```python
from build123d import *

# Parameters (mm, degrees)
SKETCH_1_R                  = 15
EXTRUDE_1_DEPTH             = 6.1
SKETCH_1_3_R                = 12.5
EXTRUDE_2_DEPTH             = 10
SKETCH_1_4_R                = 21
EXTRUDE_3_DEPTH             = 4
EXTRUDE_START               = 4
SKETCH_1_6_R                = 16.2
EXTRUDE_4_DEPTH             = 0.5
HOLE_WIZARD_M3_1_AT_2_COUNT = 2
HOLE_WIZARD_M3_1_AT_2_PITCH = 25.455844123
HOLE_WIZARD_M3_1_AT_3_COUNT = 2
HOLE_WIZARD_M3_1_AT_3_PITCH = 36
HOLE_WIZARD_M3_1_AT_4_COUNT = 2
HOLE_WIZARD_M3_1_AT_4_PITCH = 25.455844123
HOLE_WIZARD_M3_2_AT_2_COUNT = 2
HOLE_WIZARD_M3_2_AT_2_PITCH = 24
HOLE_WIZARD_M3_2_AT_3_COUNT = 2
HOLE_WIZARD_M3_2_AT_3_PITCH = 24
HOLE_WIZARD_M3_2_AT_4_COUNT = 2
HOLE_WIZARD_M3_2_AT_4_PITCH = 33.941125497
M5X0_8_1_D                  = 5
PATTERN_CIRCULAR_1_COUNT    = 6
CUT_EXTRUDE_START           = 4
SKETCH_5_R                  = 3.15
CUT_EXTRUDE_3_DEPTH         = 2.1


with BuildPart() as part:
    # ｽｹｯﾁ1 → ﾎﾞｽ - 押し出し1 (new body)
    with BuildSketch(Plane.XY):
        Circle(SKETCH_1_R)
    extrude(amount=EXTRUDE_1_DEPTH)

    # ｽｹｯﾁ1<3> → ﾎﾞｽ - 押し出し2 (add)
    with BuildSketch(Plane.XY):
        Circle(SKETCH_1_3_R)
    extrude(amount=EXTRUDE_2_DEPTH)

    # ｽｹｯﾁ1<4> → ﾎﾞｽ - 押し出し3 (add)
    with BuildSketch(Plane.XY):
        Circle(SKETCH_1_4_R)
    extrude(amount=EXTRUDE_3_DEPTH)

    # ｽｹｯﾁ1<6> → ﾎﾞｽ - 押し出し4 (add)
    with BuildSketch(Plane.XY.offset(EXTRUDE_START)):
        Circle(SKETCH_1_6_R)
    extrude(amount=EXTRUDE_4_DEPTH)

    # ｽｹｯﾁ2 → M3 丸皿ねじ用皿穴1 (revolve, cut)
    with BuildSketch(Plane(origin=(0, 18, 4), x_dir=(0, -1, 0), z_dir=(1, 0, 0))):
        Polygon((0, 0), (0, 4), (1.6, 4), (1.6, 1.55), (3.15, 0), align=None)
    hole_wizard_m3_1 = revolve(axis=Axis((0, 18, 10.35), (0, 0, -1)), mode=Mode.SUBTRACT)

    # M3 丸皿ねじ用皿穴1 at 2: M3 丸皿ねじ用皿穴1 ×2
    with Locations(*[Vector(-0.7071067811865476, -0.7071067811865476, 0) * (i * HOLE_WIZARD_M3_1_AT_2_PITCH) for i in range(1, HOLE_WIZARD_M3_1_AT_2_COUNT)]):
        add(hole_wizard_m3_1, mode=Mode.SUBTRACT)

    # M3 丸皿ねじ用皿穴1 at 3: M3 丸皿ねじ用皿穴1 ×2
    with Locations(*[(0, -i * HOLE_WIZARD_M3_1_AT_3_PITCH, 0) for i in range(1, HOLE_WIZARD_M3_1_AT_3_COUNT)]):
        add(hole_wizard_m3_1, mode=Mode.SUBTRACT)

    # M3 丸皿ねじ用皿穴1 at 4: M3 丸皿ねじ用皿穴1 ×2
    with Locations(*[Vector(0.7071067811865415, -0.7071067811865536, 0) * (i * HOLE_WIZARD_M3_1_AT_4_PITCH) for i in range(1, HOLE_WIZARD_M3_1_AT_4_COUNT)]):
        add(hole_wizard_m3_1, mode=Mode.SUBTRACT)

    # ｽｹｯﾁ8 → M3 丸皿ねじ用皿穴2 (revolve, cut)
    with BuildSketch(Plane(origin=(-12, 12, 4), x_dir=(0, -1, 0), z_dir=(1, 0, 0))):
        Polygon((0, 0), (0, 4), (1.6, 4), (1.6, 1.55), (3.15, 0), align=None)
    hole_wizard_m3_2 = revolve(axis=Axis((-12, 12, 10.35), (0, 0, -1)), mode=Mode.SUBTRACT)

    # M3 丸皿ねじ用皿穴2 at 2: M3 丸皿ねじ用皿穴2 ×2
    with Locations(*[(i * HOLE_WIZARD_M3_2_AT_2_PITCH, 0, 0) for i in range(1, HOLE_WIZARD_M3_2_AT_2_COUNT)]):
        add(hole_wizard_m3_2, mode=Mode.SUBTRACT)

    # M3 丸皿ねじ用皿穴2 at 3: M3 丸皿ねじ用皿穴2 ×2
    with Locations(*[(0, -i * HOLE_WIZARD_M3_2_AT_3_PITCH, 0) for i in range(1, HOLE_WIZARD_M3_2_AT_3_COUNT)]):
        add(hole_wizard_m3_2, mode=Mode.SUBTRACT)

    # M3 丸皿ねじ用皿穴2 at 4: M3 丸皿ねじ用皿穴2 ×2
    with Locations(*[Vector(0.7071067811865476, -0.7071067811865476, 0) * (i * HOLE_WIZARD_M3_2_AT_4_PITCH) for i in range(1, HOLE_WIZARD_M3_2_AT_4_COUNT)]):
        add(hole_wizard_m3_2, mode=Mode.SUBTRACT)

    # M5x0.8 ねじ穴1 (through all)
    with Locations(Plane.XY.offset(10)):
        with Locations((0, 0)):
            Hole(M5X0_8_1_D / 2)

    # ｽｹｯﾁ3 → M4x0.7 ねじ穴1 (revolve, cut)
    with BuildSketch(Plane(origin=(0, 9, 10), x_dir=(0, -1, 0), z_dir=(1, 0, 0))):
        Polygon((0, 0), (0, 12.491420021), (1.65, 11.5), (1.65, 0), align=None)
    m4x0_7_1 = revolve(axis=Axis((0, 9, 16.35), (0, 0, -1)), mode=Mode.SUBTRACT)

    # 円形ﾊﾟﾀｰﾝ1: M4x0.7 ねじ穴1 ×6 about axis
    pattern_circular_1_axis = Axis((0, 0, 0), (0, 0, 1))
    for i in range(1, PATTERN_CIRCULAR_1_COUNT):
        add(m4x0_7_1.rotate(pattern_circular_1_axis, i * 360 / PATTERN_CIRCULAR_1_COUNT), mode=Mode.SUBTRACT)

    # ｽｹｯﾁ5 → ｶｯﾄ - 押し出し3 (cut)
    with BuildSketch(Plane.XY.offset(CUT_EXTRUDE_START)):
        with Locations((0, 18)):
            Circle(SKETCH_5_R)
        with Locations((12, -12)):
            Circle(SKETCH_5_R)
        with Locations((18, 0)):
            Circle(SKETCH_5_R)
        with Locations((0, -18)):
            Circle(SKETCH_5_R)
        with Locations((-18, 0)):
            Circle(SKETCH_5_R)
        with Locations((-12, -12)):
            Circle(SKETCH_5_R)
        with Locations((12, 12)):
            Circle(SKETCH_5_R)
        with Locations((-12, 12)):
            Circle(SKETCH_5_R)
    extrude(amount=CUT_EXTRUDE_3_DEPTH, mode=Mode.SUBTRACT)


solid = part.part
```
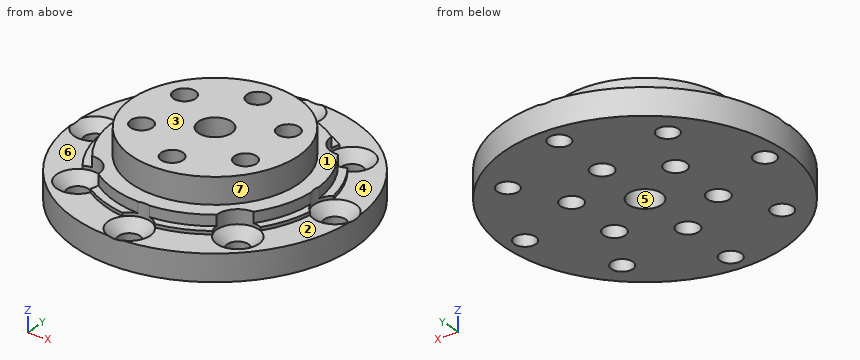
Could you check a few things on this model? Use its own coordinates, in mm. Face numbers are marked on the shaded views. A direction names the side the tool comes from. Coordinates: 2 decimals unless noted, no trailing zeros. Loops run counter-clockwise (first coordinate to the right, second up) from the corner with the lowest first, then second, coordinate; pieces in that order, holes last.
1) Will these pins go through, and if not, where does the flat tip stop? pin 1 Ø5 at (x, y) = (-12, -12) entering from +Z; pin 2 Ø6 at (x, y) = (-14.5, 10) entering from +Z; pin 3 Ø1 at (y, z) = (-7, 2) entering from -X; pin 4 Ø2.5 at (x, y) = (12, -12) entering from -Z.
Reported:
pin 1: stops at z = 3.35
pin 2: stops at z = 6.1
pin 3: stops at x = -19.97
pin 4: passes through
2) Imagine slicing it at A-A (x = 0). State how many separate pieces and enclosed holes the cut face has, and give its area (3 significant figures).
Reported:
separate pieces: 6
enclosed holes: 0
area: 181 mm2
3) Which directions (+Z, -Z, +X, -X, +Y, -Y) give clear straight access to the entire face, cutting with the end or side of a thin tool? Please do the marked faces 1, 2, 3 and 4.
Reported:
face 1: +Z
face 2: +Z, +X, -Y
face 3: +Z, +X, -X, +Y, -Y
face 4: +Z, +X, +Y
4) Thinking about a two-plate mould opening in Y: for the marked faces 5, 6 and 7, which applies, released by +Y, released by -Y, zero draft, split by the parting line, or undercut?
Reported:
face 5: undercut
face 6: zero draft
face 7: split by the parting line
5) Imagine slicing it at D-D (z = 7). List the corners of the cut face in (x, y) for me (3 decimals), and give its area (3 significant figures).
Reported:
outline: circle Ø25 at (0, 0); hole circle Ø3.3 at (-7.794, -4.5); hole circle Ø3.3 at (-7.794, 4.5); hole circle Ø5 at (0, 0); hole circle Ø3.3 at (0, -9); hole circle Ø3.3 at (0, 9); hole circle Ø3.3 at (7.794, -4.5); hole circle Ø3.3 at (7.794, 4.5)
area: 420 mm2
6) Imagine slicing it at C-C (y = -18). List the corners of the cut face in (x, z) for me, and give its area (3 significant figures).
Reported:
outline: (-10.82, 0) - (-1.6, 0) - (-1.6, 2.45) - (-3.15, 4) - (-10.82, 4) - close; (1.6, 0) - (10.82, 0) - (10.82, 4) - (3.15, 4) - (1.6, 2.45) - close
area: 71.3 mm2
7) Imagine slicing it at B-B (y = 4.5). List the corners of the cut face in (x, z) for me, and give its area (3 significant figures).
Reported:
outline: (-20.51, 0) - (-9.44, 0) - (-9.44, 10) - (-11.66, 10) - (-11.66, 6.1) - (-14.31, 6.1) - (-14.31, 4.5) - (-15.56, 4.5) - (-15.56, 4) - (-20.51, 4) - close; (-6.14, 0) - (6.14, 0) - (6.14, 10) - (-6.14, 10) - close; (9.44, 0) - (20.51, 0) - (20.51, 4) - (15.56, 4) - (15.56, 4.5) - (14.31, 4.5) - (14.31, 6.1) - (11.66, 6.1) - (11.66, 10) - (9.44, 10) - close
area: 250 mm2
8) Please list where these lines run through material, in increasing order: line 1 along X through (y, z) = (12, 1.25); line 2 along X through (y, z) = (-16, 0.75).
Reported:
line 1: x = -17.23 to -13.6, -10.4 to 10.4, 13.6 to 17.23
line 2: x = -13.6 to 13.6
